```python
from build123d import *

# Parameters (mm, degrees)
BOSS_EXTRUDE1_DEPTH      = 5
BOSS_EXTRUDE1_DEPTH_BACK = 105
SKETCH5_W                = 32
SKETCH5_H                = 95
CUT_EXTRUDE1_DEPTH       = 100
SKETCH7_R                = 5
CUT_EXTRUDE2_DEPTH       = 40
CUT_EXTRUDE2_DEPTH_BACK  = 113
CUT_EXTRUDE4_DEPTH       = 234
CUT_EXTRUDE4_DEPTH_BACK  = 234


with BuildPart() as part:
    # Sketch2 → Revolve2 (revolve)
    with BuildSketch(Plane(origin=(0, 0, 0), x_dir=(0, 0, -1), z_dir=(1, 0, 0)), mode=Mode.PRIVATE) as revolve2_sk:
        Polygon((15.054954353, -7.686097714), (-68.645045647, -7.686097714), (-68.645045647, 2.203003026), (-66.645045647, 4.813902286), (-13.645045647, 4.813902286), (-13.645045647, 12.313902286), (11.354954353, 12.313902286), (15.054954353, 15.806805515), align=None)
    revolve(revolve2_sk.sketch.rotate(Axis((0, -7.686097714, -15.054954353), (0, 0, 1)), 90), axis=Axis((0, -7.686097714, -15.054954353), (0, 0, 1)))

    # 3DSketch2 → Boss-Extrude1 (add, two sides)
    with BuildSketch(Plane(origin=(26.001222768, 22.321847461, -19.965853613), x_dir=(-0.6549305384178419, -0.7556890827898176, 0), z_dir=(0, 0, 1))) as boss_extrude1_sk:
        Polygon((0, 0), (34.056387998, -39.295832305), (79.397732965, 0), (45.341344967, 39.295832305), align=None)
    extrude(amount=BOSS_EXTRUDE1_DEPTH)
    extrude(boss_extrude1_sk.sketch, amount=-BOSS_EXTRUDE1_DEPTH_BACK)

    # Sketch5 → Cut-Extrude1 (cut)
    with BuildSketch(Plane(origin=(0, 22.321847461, 0), x_dir=(1, 0, 0), z_dir=(0, 1, 0))):
        with Locations((0.001222768, 77.465853613)):
            Rectangle(SKETCH5_W, SKETCH5_H)
    extrude(amount=-CUT_EXTRUDE1_DEPTH, mode=Mode.SUBTRACT)

    # Sketch7 → Cut-Extrude2 (cut, two sides)
    with BuildSketch(Plane(origin=(26.001222768, 0, 0), x_dir=(0, 0, -1), z_dir=(1, 0, 0))) as cut_extrude2_sk:
        with Locations(Location((76.965853613, -7.678152539, 0), (0, 0, 180))):
            Circle(SKETCH7_R)
        with Locations(Location((108.965853613, -7.678152539, 0), (0, 0, 180))):
            Circle(SKETCH7_R)
    extrude(amount=CUT_EXTRUDE2_DEPTH, mode=Mode.SUBTRACT)
    extrude(cut_extrude2_sk.sketch, amount=-CUT_EXTRUDE2_DEPTH_BACK, mode=Mode.SUBTRACT)

    # Sketch8 → Cut-Extrude4 (cut, two sides)
    with BuildSketch(Plane(origin=(26.001222768, 0, 0), x_dir=(0, 0, -1), z_dir=(1, 0, 0))) as cut_extrude4_sk:
        with BuildLine():
            Line((124.965853613, -7.678152493), (124.965853613, 22.321847461))
            Line((124.965853613, 22.321847461), (94.965853613, 22.321847461))
            ThreePointArc((94.965853613, 22.321847461), (116.179057032, 13.535050913), (124.965853613, -7.678152493))
        make_face()
        with BuildLine():
            Line((124.965853613, -37.678152539), (124.965853613, -7.678152493))
            ThreePointArc((124.965853613, -7.678152493), (116.179057065, -28.891355958), (94.965853613, -37.678152539))
            Line((94.965853613, -37.678152539), (124.965853613, -37.678152539))
        make_face()
    extrude(amount=CUT_EXTRUDE4_DEPTH, mode=Mode.SUBTRACT)
    extrude(cut_extrude4_sk.sketch, amount=-CUT_EXTRUDE4_DEPTH_BACK, mode=Mode.SUBTRACT)


solid = part.part
```
Model file for the job. Use its own axes, mm. A direction names the side the tool comes from. Give positions to 0.01 mm unless a question says otherwise; leave off trailing zeros. Write each loop counter-clockwise with the first axis right and the second up, starting at its lowest first coordinate (ties: lowest second). Pieces come first, ordered by that corner, then holes. Notation, with made-up numbers: M 74,54 L 108,54 A27 ccw 108,75 Z; hole C 57,-10.5 d1. An arc over 180 degrees is marked long. Use a Markdown table: item, result.
1) Cut at A-A (z = -47). List the corners of the cut face in (x, y).
Responses:
| item | result |
|---|---|
| outline | M -26,-37.68 L -16,-37.68 L -16,22.32 L -26,22.32 Z; M 16,-37.68 L 26,-37.68 L 26,22.32 L 16,22.32 Z |
2) Tool access for faces 4 (the flat face through (0, -8, 68.645)), 5 (the flat face through (0, -7, -29.966)), 6 (the flat face through (-21, 3, -14.966)): list every direction of +Z, -Z, +X, -X, +Y, -Y with a clear straight run to the whole face (end or side of a thin tool).
Responses:
| item | result |
|---|---|
| face 4 | +Z, +X, -X, +Y, -Y |
| face 5 | -Z, +Y, -Y |
| face 6 | +Z |
3) Cut at B-B (x = 0). List the corners of the cut face in (y, z), and give its area (3 significant figures).
Responses:
| item | result |
|---|---|
| outline | M -37.68,-29.97 L 22.32,-29.97 L 22.32,-14.97 L 15.72,-14.97 L 12.31,-11.35 L 12.31,13.65 L 4.81,13.65 L 4.81,66.65 L 2.2,68.65 L -17.58,68.65 L -20.19,66.65 L -20.19,13.65 L -27.69,13.65 L -27.69,-11.35 L -31.09,-14.97 L -37.68,-14.97 Z |
| area | 3,430 mm2 |
4) Pull direction Z, two halves, no side cores. Call faces 1 (the conical face through (2.631, -27.727, -11.581)), 2 (the cylindrical face through (-20.93, -5.76, -104.35)), 3 (the flat face through (16.001, -14, -77)): +Z half, -Z half, draft (parallel to the pull), parting line (faces both ways), or undercut.
Responses:
| item | result |
|---|---|
| face 1 | +Z half |
| face 2 | undercut |
| face 3 | draft |
5) Pin check, flat tips, straight feed: pin 1 (11.5 mm diameter, centred on y = -7.68, z = -108.97, fed in from +X); pin 2 (1 mm diameter, centred on x = 10, z = -10.5, fed in from -Y); pin 3 (9.5 mm diameter, centred on x = 1.5, y = -12, fed in from -Z); pin 4 (5 mm diameter, centred on x = -6, y = -30, fed in from +Z). Stop position of each tip, or through.
Responses:
| item | result |
|---|---|
| pin 1 | stops at x = 26 |
| pin 2 | stops at y = -25.29 |
| pin 3 | stops at z = -29.97 |
| pin 4 | stops at z = -12 |
6) Cut at D-D (z = 25). List the corners of the cut face in (x, y), and give its area (3 significant figures).
Responses:
| item | result |
|---|---|
| outline | C 0,-7.69 d25 |
| area | 491 mm2 |
7) Drill centre lines: line 1 (X direction, y = -13, z = -66); line 2 (Z direction, x = 12.5, y = 16); line 3 (Z direction, x = 7.5, y = 8.5). Where is each one in solid material? Low to high. Write a range as from..to.
Responses:
| item | result |
|---|---|
| line 1 | x = -26..-16, 16..26 |
| line 2 | z = -29.97..-14.97 |
| line 3 | z = -29.97..13.65 |
8) Cut at C-C (z = -75). List the corners of the cut face in (x, y), and give its area (3 significant figures).
Responses:
| item | result |
|---|---|
| outline | M -26,-37.68 L -16,-37.68 L -16,-12.28 L -26,-12.28 Z; M -26,-3.08 L -16,-3.08 L -16,22.32 L -26,22.32 Z; M 16,-37.68 L 26,-37.68 L 26,-12.28 L 16,-12.28 Z; M 16,-3.08 L 26,-3.08 L 26,22.32 L 16,22.32 Z |
| area | 1,020 mm2 |
